```python
from build123d import *

# Parameters (mm, degrees)
SKETCH_1_R          = 5
EXTRUDE_1_DEPTH     = 35
SKETCH_2_R          = 6
EXTRUDE_2_DEPTH     = 3
SKETCH_3_R          = 15
SKETCH_3_R_2        = 2
EXTRUDE_3_DEPTH     = 3
CUT_EXTRUDE_1_DEPTH = 19
SKETCH_5_R          = 1.5
CUT_EXTRUDE_2_DEPTH = 48.613023428
SKETCH_6_R          = 2.5
CUT_EXTRUDE_3_DEPTH = 47.16275555
SKETCH_7_R          = 3.5
CUT_EXTRUDE_4_DEPTH = 3


with BuildPart() as part:
    # 草图1 → 凸台-拉伸1 (new body)
    with BuildSketch(Plane.XY):
        Circle(SKETCH_1_R)
    extrude(amount=EXTRUDE_1_DEPTH)

    # 草图2 → 凸台-拉伸2 (add)
    with BuildSketch(Plane.XY.offset(35)):
        Circle(SKETCH_2_R)
    extrude(amount=EXTRUDE_2_DEPTH)

    # 草图3 → 凸台-拉伸3 (add)
    with BuildSketch(Plane.XY.offset(38)):
        Circle(SKETCH_3_R)
        with Locations((0, 10)):
            Circle(SKETCH_3_R_2, mode=Mode.SUBTRACT)
        with Locations((10, 0)):
            Circle(SKETCH_3_R_2, mode=Mode.SUBTRACT)
        with Locations((0, -10)):
            Circle(SKETCH_3_R_2, mode=Mode.SUBTRACT)
        with Locations((-10, 0)):
            Circle(SKETCH_3_R_2, mode=Mode.SUBTRACT)
        with Locations((7.071067812, 7.071067812)):
            Circle(SKETCH_3_R_2, mode=Mode.SUBTRACT)
        with Locations((7.071067812, -7.071067812)):
            Circle(SKETCH_3_R_2, mode=Mode.SUBTRACT)
        with Locations((-7.071067812, -7.071067812)):
            Circle(SKETCH_3_R_2, mode=Mode.SUBTRACT)
        with Locations((-7.071067812, 7.071067812)):
            Circle(SKETCH_3_R_2, mode=Mode.SUBTRACT)
    extrude(amount=EXTRUDE_3_DEPTH)

    # 草图4 → 切除-拉伸1 (cut)
    with BuildSketch(Plane(origin=(0, 0, 0), x_dir=(-1, 0, 0), z_dir=(0, 0, -1))):
        with BuildLine():
            Line((-3, 4), (3, 4))
            ThreePointArc((3, 4), (0, 5), (-3, 4))
        make_face()
        with BuildLine():
            Line((-3, -4), (3, -4))
            ThreePointArc((3, -4), (0, -5), (-3, -4))
        make_face()
    extrude(amount=-CUT_EXTRUDE_1_DEPTH, mode=Mode.SUBTRACT)

    # 草图5 → 切除-拉伸2 (cut, through all)
    with BuildSketch(Plane(origin=(0, 4, 0), x_dir=(1, 0, 0), z_dir=(0, 1, 0))):
        with Locations(Location((0, -16.5, 0), (0, 0, 270))):
            Circle(SKETCH_5_R)
    extrude(amount=-CUT_EXTRUDE_2_DEPTH, mode=Mode.SUBTRACT)

    # 草图6 → 切除-拉伸3 (cut, through all)
    with BuildSketch(Plane(origin=(0, 0, 0), x_dir=(-1, 0, 0), z_dir=(0, 0, -1))):
        Circle(SKETCH_6_R)
    extrude(amount=-CUT_EXTRUDE_3_DEPTH, mode=Mode.SUBTRACT)

    # 草图7 → 切除-拉伸4 (cut)
    with BuildSketch(Plane.XY.offset(41)):
        Circle(SKETCH_7_R)
    extrude(amount=-CUT_EXTRUDE_4_DEPTH, mode=Mode.SUBTRACT)


solid = part.part
```
Read the model definition and answer for the solid it produces. Units are mm, in the model's axes. A direction names the side the tool comes from. Give positions to 0.01 mm unless a question says otherwise; leave off trailing zeros. Order: outer loops, then holes, each group sorted by start corner. A loop starts at its lowest first (then second) coordinate and runs counter-clockwise, first axis right, second up.
(1) Given pin 1 (3 mm diameter, centred on x = 0, z = 9.5, fed in from +Y); pin 2 (10 mm diameter, centred on x = -10, y = 9.5, fed in from -Z); pin 3 (1 mm diameter, centred on x = 7, z = 32.5, fed in from -Y); pin 4 (4 mm diameter, centred on x = 6.5, z = 11, fed in from +Y), each flat-ended and moving along its own axis, determine where each tip first touches the part or whether it passes through.
(2) Find section B-B (y = 0). Give the vertices of the cut face in (x, z), plus the area to 3 significant figures.
(3) Straight lines are drawn through the part: L1, parallel to Y at x = 0, z = 39.9; L2, parallel to X at y = 8.5, z = 39; L3, parallel to Z at x = -5.75, y = -3.75. For each, find the intervals that lie inside material, in ascending order.
(4) For a pull along Y with two mould halves and no side action, classify faces 1 (the flat face through (0, 4, 9)), 2 (the flat face through (0, 4.4, 19)), 3 (the cylindrical face through (8.146, -5.385, 39.479)) as released by +Y, released by -Y, zero draft, split by the parting line, or undercut.
(5) Find section D-D (y = -10). Give the vertices of the cut face in (x, z), plus the area to 3 significant figures.
(6) Find section A-A (z = 16.5). Give the vertices of the cut face in (x, y).
(7) For faces 4 (the cylindrical face through (-6, -5.38, 39.48)), 5 (the cylindrical face through (-5, 0, 21)), 6 (the flat face through (2, -2, 38)), determine the directions among +Z, -Z, +X, -X, +Y, -Y from which every point of the face is accessible in a straight line to the end or side of a thin tool.
(8) Find section C-C (x = -7). Give the vertices of the cut face in (y, z), plus the area to 3 significant figures.
Result sheet:
1. pin 1: stops at y = 4
1. pin 2: stops at z = 38
1. pin 3: passes through
1. pin 4: stops at y = 2.18
2. outline: (-15, 38) - (-12, 38) - (-12, 41) - (-15, 41) - close; (-8, 38) - (-6, 38) - (-6, 35) - (-5, 35) - (-5, 0) - (-2.5, 0) - (-2.5, 38) - (-3.5, 38) - (-3.5, 41) - (-8, 41) - close; (2.5, 0) - (5, 0) - (5, 35) - (6, 35) - (6, 38) - (8, 38) - (8, 41) - (3.5, 41) - (3.5, 38) - (2.5, 38) - close; (12, 38) - (15, 38) - (15, 41) - (12, 41) - close
2. area: 241 mm2
3. L1: y = -15 to -12, -8 to -3.5, 3.5 to 8, 12 to 15
3. L2: x = -12.36 to -8.47, -5.67 to -1.32, 1.32 to 5.67, 8.47 to 12.36
3. L3: z = 38 to 41
4. face 1: released by +Y
4. face 2: zero draft
4. face 3: undercut
5. outline: (-11.18, 38) - (-2, 38) - (-2, 41) - (-11.18, 41) - close; (2, 38) - (11.18, 38) - (11.18, 41) - (2, 41) - close
5. area: 55.1 mm2
6. outline: (-3, -4) - (-1.5, -4) - (-1.5, -2) arc R2.5 cw to (-1.5, 2) - (-1.5, 4) - (-3, 4) arc R5 ccw to start; (1.5, -4) - (3, -4) arc R5 ccw to (3, 4) - (1.5, 4) - (1.5, 2) arc R2.5 cw to (1.5, -2) - close
7. face 4: +Z, -Z
7. face 5: -Z
7. face 6: +Z
8. outline: (-13.27, 38) - (-9.07, 38) - (-9.07, 41) - (-13.27, 41) - close; (-5.07, 38) - (5.07, 38) - (5.07, 41) - (-5.07, 41) - close; (9.07, 38) - (13.27, 38) - (13.27, 41) - (9.07, 41) - close
8. area: 55.6 mm2
